```python
from build123d import *

# Parameters (mm, degrees)
EXTRUDE_1_DEPTH     = 240
SKETCH_2_R          = 5
CUT_EXTRUDE_1_DEPTH = 10
SKETCH_3_R          = 5
CUT_EXTRUDE_2_DEPTH = 10


with BuildPart() as part:
    # Эскиз1 → Вытянуть-Тонкостенный1 (new body)
    with BuildSketch(Plane(origin=(0, 0, 0), x_dir=(1, 0, 0), z_dir=(0, 1, 0))):
        Polygon((0, 50), (0, 0), (50, 0), (50, 4), (4, 4), (4, 50), align=None)
    extrude(amount=EXTRUDE_1_DEPTH)

    # Эскиз2 → Вырез-Вытянуть1 (cut)
    with BuildSketch(Plane.XY):
        with Locations((27, 225)):
            Circle(SKETCH_2_R)
        with Locations((27, 125)):
            Circle(SKETCH_2_R)
        with Locations((27, 25)):
            Circle(SKETCH_2_R)
    extrude(amount=-CUT_EXTRUDE_1_DEPTH, mode=Mode.SUBTRACT)

    # Эскиз3 → Вырез-Вытянуть2 (cut)
    with BuildSketch(Plane.ZY):
        with Locations((-23, 225)):
            Circle(SKETCH_3_R)
        with Locations((-23, 125)):
            Circle(SKETCH_3_R)
        with Locations((-23, 25)):
            Circle(SKETCH_3_R)
    extrude(amount=-CUT_EXTRUDE_2_DEPTH, mode=Mode.SUBTRACT)


solid = part.part
```
Geometry: final body of the model. Coordinates: model frame, mm. A direction names the side the tool comes from. Coordinates: 2 decimals unless noted, no trailing zeros. Order: outer loops, then holes, each group sorted by start corner. A loop starts at its lowest first (then second) coordinate and runs counter-clockwise, first axis right, second up. Notation, with made-up numbers: (12, -13.5) - (34, -13.5) arc R7 cw to (34, -5.5) - close; hole circle Ø1 at (65.25, -16.5). An arc over 180 degrees is marked (long way). Return JSON: item names as keys, results as strings. Group by question number.
1. Cut plane A-A (z = -23). Output: boundary loops of the cut face in (x, y).
2. Cut plane C-C (y = 225). Output: boundary loops of the cut face in (x, z), plus the area to 3 significant figures.
3. Cut plane D-D (y = 52). Output: boundary loops of the cut face in (x, z).
4. Cut plane B-B (x = 27). Output: boundary loops of the cut face in (y, z), plus the area to 3 significant figures.
5. Pull-direction query (X, two-part tool) for faces 3 (the face through (25.92, 20.12, -1.97)), 4 (the face through (4, 118, -27)), 5 (the face through (22, 125, -2)), 6 (the face through (3, 0, -14)); classes: pulls with the +X half, pulls with the -X half, needs draft (parallel to the pull), parting line crosses it, or undercut.
6. Material intervals for line 1 along Y through (x, z) = (2, -23); line 2 along X through (y, z) = (123.5, -37); line 3 along Z through (x, y) = (35, 56.5), sorted ascending. Write a range as [from, to].
7. Pin query (flat end, axial travel): pin 1 (13 mm diameter, centred on x = 27, y = 25, fed in from -Z); pin 2 (8 mm diameter, centred on x = 24, y = 94, fed in from +Z); pin 3 (6 mm diameter, centred on y = 25, z = -23, fed in from -X); pin 4 (13 mm diameter, centred on y = 225, z = -23, fed in from +X). Return the tip coordinate at first contact, or that it passes through.
8. Set-up query: faces 1 (the face through (26.349, 229.957, -1.972)), 2 (the face through (27, 118, -4)). Return all of +Z, -Z, +X, -X, +Y, -Y with unobstructed straight access to the full face (end or side cutting, diameter ignored); none if empty.
Resolved:
{
 "1": {"outline": "(0, 0) - (4, 0) - (4, 20) - (0, 20) - close; (0, 30) - (4, 30) - (4, 120) - (0, 120) - close; (0, 130) - (4, 130) - (4, 220) - (0, 220) - close; (0, 230) - (4, 230) - (4, 240) - (0, 240) - close"},
 "2": {"outline": "(0, -50) - (4, -50) - (4, -28) - (0, -28) - close; (0, -18) - (4, -18) - (4, -4) - (22, -4) - (22, 0) - (0, 0) - close; (32, -4) - (50, -4) - (50, 0) - (32, 0) - close", "area": "304 mm²"},
 "3": {"outline": "(0, -50) - (4, -50) - (4, -4) - (50, -4) - (50, 0) - (0, 0) - close"},
 "4": {"outline": "(0, -4) - (20, -4) - (20, 0) - (0, 0) - close; (30, -4) - (120, -4) - (120, 0) - (30, 0) - close; (130, -4) - (220, -4) - (220, 0) - (130, 0) - close; (230, -4) - (240, -4) - (240, 0) - (230, 0) - close", "area": "840 mm²"},
 "5": {"face 3": "undercut", "face 4": "pulls with the +X half", "face 5": "undercut", "face 6": "needs draft"},
 "6": {"line 1": "y = [0, 20], [30, 120], [130, 220], [230, 240]", "line 2": "x = [0, 4]", "line 3": "z = [-4, 0]"},
 "7": {"pin 1": "stops at z = -4", "pin 2": "stops at z = 0", "pin 3": "passes through", "pin 4": "stops at x = 4"},
 "8": {"face 1": "+Z, -Z", "face 2": "-Z, +X, +Y, -Y"}
}
